```python
from build123d import *

# Parameters (mm, degrees)
CYLINDER003001001005001001_R     = 3.5
CYLINDER003001001005001001_DEPTH = 2
CYLINDER003001001004002_R        = 1
CYLINDER003001001004002_DEPTH    = 5
CYLINDER003001001004001001_R     = 1
CYLINDER003001001004001001_DEPTH = 5
CYLINDER003001001005001_R        = 6.5
CYLINDER003001001005001_DEPTH    = 2
BOX002_W                         = 10
BOX002_H                         = 6
BOX002_DEPTH                     = 2
CYLINDER003001001004_R           = 2
CYLINDER003001001004_DEPTH       = 3
CYLINDER003001001004001_R        = 2
CYLINDER003001001004001_DEPTH    = 3
CYLINDER003001001005_R           = 15
CYLINDER003001001005_DEPTH       = 2
CUT002_ROLL_ANGLE                = 180
CUT002_PLACEMENT_ANGLE           = -90.233929


with BuildPart() as cylinder013:
    # Cylinder003001001005001001 → Cylinder003001001005001001 (new body)
    with BuildSketch(Plane(origin=(12, 6, 21), x_dir=(1, 0, 0), z_dir=(0, 0, 1))):
        Circle(CYLINDER003001001005001001_R)
    extrude(amount=CYLINDER003001001005001001_DEPTH)


with BuildPart() as cylinder014:
    # Cylinder003001001004002 → Cylinder003001001004002 (new body)
    with BuildSketch(Plane(origin=(-2.5, 6, 16.4), x_dir=(1, 0, 0), z_dir=(0, 0, 1))):
        Circle(CYLINDER003001001004002_R)
    extrude(amount=CYLINDER003001001004002_DEPTH)


with BuildPart() as cylinder015:
    # Cylinder003001001004001001 → Cylinder003001001004001001 (new body)
    with BuildSketch(Plane(origin=(25.5, 6, 16.4), x_dir=(1, 0, 0), z_dir=(0, 0, 1))):
        Circle(CYLINDER003001001004001001_R)
    extrude(amount=CYLINDER003001001004001001_DEPTH)


with BuildPart() as fusion009:
    # Cylinder003001001005001 → Cylinder003001001005001 (new body)
    with BuildSketch(Plane(origin=(6, 6, 21), x_dir=(1, 0, 0), z_dir=(0, 0, 1))):
        Circle(CYLINDER003001001005001_R)
    extrude(amount=CYLINDER003001001005001_DEPTH)

    # Fusion009: union Cylinder013, Cylinder014, Cylinder015
    add(cylinder013.part)
    add(cylinder014.part)
    add(cylinder015.part)


with BuildPart() as box002:
    # Box002 → Box002 (new body)
    with BuildSketch(Plane(origin=(18, 3, 21), x_dir=(1, 0, 0), z_dir=(0, 0, 1))):
        with Locations((5, 3)):
            Rectangle(BOX002_W, BOX002_H)
    extrude(amount=BOX002_DEPTH)


with BuildPart() as cylinder003001001004:
    # Cylinder003001001004 → Cylinder003001001004 (new body)
    with BuildSketch(Plane(origin=(-2.5, 6, 18.4), x_dir=(1, 0, 0), z_dir=(0, 0, 1))):
        Circle(CYLINDER003001001004_R)
    extrude(amount=CYLINDER003001001004_DEPTH)


with BuildPart() as cylinder010:
    # Cylinder003001001004001 → Cylinder003001001004001 (new body)
    with BuildSketch(Plane(origin=(25.5, 6, 18.4), x_dir=(1, 0, 0), z_dir=(0, 0, 1))):
        Circle(CYLINDER003001001004001_R)
    extrude(amount=CYLINDER003001001004001_DEPTH)


with BuildPart() as guide1:
    # Cylinder003001001005 → Cylinder003001001005 (new body)
    with BuildSketch(Plane(origin=(6, 6, 21), x_dir=(1, 0, 0), z_dir=(0, 0, 1))):
        Circle(CYLINDER003001001005_R)
    extrude(amount=CYLINDER003001001005_DEPTH)

    # Fusion008: union Box002, Cylinder003001001004, Cylinder010
    add(box002.part)
    add(cylinder003001001004.part)
    add(cylinder010.part)

    # Cut002: cut Fusion009
    add(fusion009.part, mode=Mode.SUBTRACT)


with BuildPart() as guide1_1:
    # Cut002 roll: moved
    add(guide1.part.rotate(Axis((0, 0, 0), (1, 0, 0)), CUT002_ROLL_ANGLE))


with BuildPart() as guide1_2:
    # Cut002 placement: moved
    add(guide1_1.part.moved(Location((80, 36, 62))).rotate(Axis((80, 36, 62), (0, 0, 1)), CUT002_PLACEMENT_ANGLE))


solid = guide1_2.part
```
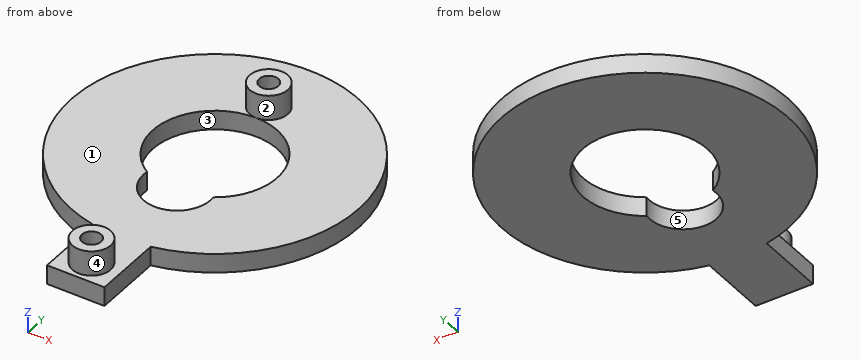
Can you work these out from the model? Positions are in its coordinate system, mm. Face numbers are marked on the shaded views. A direction names the side the tool comes from. Round coordinates to 2 decimals unless told otherwise and drop trailing zeros. Loops run counter-clockwise (first coordinate to the right, second up) from the corner with the lowest first, then second, coordinate; pieces in that order, holes last.
Item 1: Suppose I cut it at C-C, the plane z = 41.6. Write out the boundary of the cut face in (x, y).
Item 2: Suppose I cut it at B-B, the plane x = 69.75. Write out the boundary of the cut face in (y, z).
Item 3: Which directions (+Z, -Z, +X, -X, +Y, -Y) give clear straight access to the entire face, cutting with the end or side of a thin tool? Please do the marked faces 4 and 5.
Item 4: Suppose I cut it at A-A, the plane y = 21. Write out the boundary of the cut face in (x, z).
Item 5: Please list where these lines run through material, in increasing order: L1, parallel to Z at x = 69, y = 36; L2, parallel to X at y = 10, z = 42.75; L3, parallel to Y at x = 71.25, z = 40.3.
Item 6: If we mould it in two halves opening along X, with no side actions, what happens to the marked faces 1, 2 and 3? For each: +X half, -X half, draft (parallel to the pull), parting line (faces both ways), or undercut.
Item 7: Suppose I cut it at D-D, the plane z = 39.5. Write out the boundary of the cut face in (x, y), then the cut area to 3 significant figures.
Item 8: Will these pins go through, and if not, where does the flat tip stop? pin 1 Ø10 at (x, y) = (85.5, 13.5) entering from +Z; pin 2 Ø2 at (x, z) = (78.5, 40) entering from +Y; pin 3 Ø1.6 at (x, y) = (74.01, 38.52) entering from +Z; pin 4 Ø1.5 at (x, z) = (63.5, 39.5) entering from -Y.
Reported:
1. outline: circle Ø4 at (73.9, 10.52); circle Ø4 at (74.01, 38.52); hole circle Ø2 at (73.9, 10.52); hole circle Ø2 at (74.01, 38.52)
2. outline: (15.63, 39) - (25.09, 39) - (25.09, 41) - (15.63, 41) - close; (34.96, 39) - (44.42, 39) - (44.42, 41) - (34.96, 41) - close
3. face 4: +Z
3. face 5: +Z, -Z
4. outline: (61.99, 39) - (72.19, 39) - (72.19, 41) - (61.99, 41) - close; (75.71, 39) - (85.96, 39) - (85.96, 41) - (75.71, 41) - close
5. L1: z = 39 to 41
5. L2: x = 71.97 to 73.04, 74.75 to 75.83
5. L3: y = 8.04 to 21.8, 35.93 to 44.77
6. face 1: draft
6. face 2: parting line
6. face 3: undercut
7. outline: (70.89, 8.04) - (76.89, 8.01) - (76.92, 15.32) arc R15 ccw (long way) to (70.92, 15.34) - close; hole (70.49, 24.54) arc R3.5 ccw (long way) to (77.42, 24.51) arc R6.5 ccw (long way) to start
7. area: 599 mm2
8. pin 1: passes through
8. pin 2: stops at y = 44.6
8. pin 3: stops at z = 40.6
8. pin 4: stops at y = 18.6
